```python
from build123d import *

# Parameters (mm, degrees)
CROQUIS1_W              = 730
CROQUIS1_H              = 180
SALIENTE_EXTRUIR1_DEPTH = 15
CROQUIS2_R              = 2
CORTAR_EXTRUIR1_DEPTH   = 10
CROQUIS3_R              = 22.5
CORTAR_EXTRUIR2_DEPTH   = 15
CROQUIS4_R              = 4
CORTAR_EXTRUIR3_DEPTH   = 15


with BuildPart() as part:
    # Croquis1 → Saliente-Extruir1 (new body)
    with BuildSketch(Plane.XY):
        Rectangle(CROQUIS1_W, CROQUIS1_H)
    extrude(amount=SALIENTE_EXTRUIR1_DEPTH)

    # Croquis2 → Cortar-Extruir1 (cut)
    with BuildSketch(Plane.XY.offset(15)):
        with Locations((-340, -25)):
            Circle(CROQUIS2_R)
        with Locations((0, -65)):
            Circle(CROQUIS2_R)
        with Locations((0, -45)):
            Circle(CROQUIS2_R)
        with Locations((-320, -25)):
            Circle(CROQUIS2_R)
        with Locations((340, -25)):
            Circle(CROQUIS2_R)
        with Locations((320, -25)):
            Circle(CROQUIS2_R)
    extrude(amount=-CORTAR_EXTRUIR1_DEPTH, mode=Mode.SUBTRACT)

    # Croquis3 → Cortar-Extruir2 (cut)
    with BuildSketch(Plane.XY.offset(15)):
        Circle(CROQUIS3_R)
    extrude(amount=-CORTAR_EXTRUIR2_DEPTH, mode=Mode.SUBTRACT)

    # Croquis4 → Cortar-Extruir3 (cut)
    with BuildSketch(Plane(origin=(0, 0, 0), x_dir=(-1, 0, 0), z_dir=(0, 0, -1))):
        with Locations((-305, -50)):
            Circle(CROQUIS4_R)
    extrude(amount=-CORTAR_EXTRUIR3_DEPTH, mode=Mode.SUBTRACT)


solid = part.part
```
Geometry check sheet. Reference: the model listing, model coordinates, mm. Coordinates: 2 decimals unless noted, no trailing zeros. Write each loop counter-clockwise with the first axis right and the second up, starting at its lowest first coordinate (ties: lowest second). Pieces come first, ordered by that corner, then holes. Notation, with made-up numbers: M 11.25,21 L 65.25,21 A12 ccw 65.25,36 Z; hole C -17,71 d2. An arc over 180 degrees is marked long. One line per item, written item: value. Start each with the question number.
(1) Release check for a two-part mould opening along Y. For faces 1 (the face through (10.382, -19.961, 7.605)), 2 (the face through (-365, -1, 7)), 3 (the face through (-5, 90, 7)) record: released by +Y, released by -Y, zero draft, split by the parting line, or undercut.
(2) Depth check by flat-ended pin: pin 1 (2 mm diameter, centred on x = -320.5, y = -24.5, fed in from +Z). Enter the tip coordinate at first touch or a pass-through.
(3) Scan lines: line 1 along Y through (x, z) = (340, 8.5); line 2 along X through (y, z) = (11.5, 4); line 3 along X through (y, z) = (15.5, 5). Record each from-to range of solid material in increasing order. Write a range as [from, to].
(4) Sectioned sample at A-A, the plane y = -9. Enter the section's corners in (x, z).
Filled sheet:
1. face 1: undercut
1. face 2: zero draft
1. face 3: released by +Y
2. pin 1: z = 5
3. line 1: [-90, -27], [-23, 90]
3. line 2: [-365, -19.34], [19.34, 365]
3. line 3: [-365, -16.31], [16.31, 365]
4. outline: M -365,0 L -20.62,0 L -20.62,15 L -365,15 Z; M 20.62,0 L 365,0 L 365,15 L 20.62,15 Z
